from build123d import *

# Parameters (mm, degrees)
MAIN_DEPTH  = 4.7625
SKETCH2_R   = 6.35
SKETCH2_R_2 = 23.8125
HOLES_DEPTH = 67.238901193


with BuildPart() as part:
    # Sketch1 → Main (new body)
    with BuildSketch(Plane.XY):
        with BuildLine():
            Line((12.894196685, 47.360416667), (30.946072045, 22.225))
            ThreePointArc((30.946072045, 22.225), (38.1, 0), (30.946072045, -22.225))
            Line((30.946072045, -22.225), (12.894196685, -47.360416667))
            ThreePointArc((12.894196685, -47.360416667), (0, -53.975), (-12.894196685, -47.360416667))
            Line((-12.894196685, -47.360416667), (-30.946072045, -22.225))
            ThreePointArc((-30.946072045, -22.225), (-38.1, 0), (-30.946072045, 22.225))
            Line((-30.946072045, 22.225), (-12.894196685, 47.360416667))
            ThreePointArc((-12.894196685, 47.360416667), (0, 53.975), (12.894196685, 47.360416667))
        make_face()
    extrude(amount=MAIN_DEPTH)

    # Sketch2 → Holes (cut, through all)
    with BuildSketch(Plane.XY.offset(4.7625)):
        with Locations((0, 38.1)):
            Circle(SKETCH2_R)
        with Locations((0, -38.1)):
            Circle(SKETCH2_R)
        Circle(SKETCH2_R_2)
    extrude(amount=-HOLES_DEPTH, mode=Mode.SUBTRACT)


solid = part.part
The listing builds one solid part. Answer for the finished solid, in the listing's coordinates (mm). Give positions to 0.01 mm unless a question says otherwise; leave off trailing zeros. Order: outer loops, then holes, each group sorted by start corner. A loop starts at its lowest first (then second) coordinate and runs counter-clockwise, first axis right, second up. Notation, with made-up numbers: (61.25, 10.25) -> (69.25, 10.25) arc R25 ccw to (69.25, 22.25) -> close; hole circle Ø4 at (89.25, 59). An arc over 180 degrees is marked (long way). Put each result on its own line as item: value.
Item 1: A cutting plane is placed at D-D on x = 20. Give the vertices of the cut face in (y, z).
Established:
outline: (-37.47, 0) -> (-12.92, 0) -> (-12.92, 4.76) -> (-37.47, 4.76) -> close; (12.92, 0) -> (37.47, 0) -> (37.47, 4.76) -> (12.92, 4.76) -> close
Item 2: A cutting plane is placed at A-A on y = 0. Give the vertices of the cut face in (x, z).
Established:
outline: (-38.1, 0) -> (-23.81, 0) -> (-23.81, 4.76) -> (-38.1, 4.76) -> close; (23.81, 0) -> (38.1, 0) -> (38.1, 4.76) -> (23.81, 4.76) -> close
Item 3: Straight lines are drawn through the part: line 1 (X direction, y = -11, z = 2.55); line 2 (Y direction, x = -21.5, z = 2); line 3 (Y direction, x = -8, z = 1.1). For each, find the intervals that lie inside material, in ascending order.
Established:
line 1: x = -36.48 to -21.12, 21.12 to 36.48
line 2: y = -35.38 to -10.24, 10.24 to 35.38
line 3: y = -51.81 to -22.43, 22.43 to 51.81
Item 4: Given P1, Ø10, axis at x = 0, y = -38.1, coming from the +Z side; P2, Ø1.5, axis at x = -20, z = 4, coming from the +Y side, each flat-ended and moving along its own axis, determine where each tip first touches the part or whether it passes through.
Established:
P1: passes through
P2: stops at y = 38.51
Item 5: For a pull along Y with two mould halves and no side action, classify faces 1 (the face through (1, 25, 4.762)), 2 (the face through (-18.897, -14.49, 2.415)), 3 (the face through (-38.1, -0.3, 2.3)), 4 (the face through (21.794, 34.969, 2.348)) as released by +Y, released by -Y, zero draft, split by the parting line, or undercut.
Established:
face 1: zero draft
face 2: undercut
face 3: split by the parting line
face 4: released by +Y
Item 6: A cutting plane is placed at B-B on x = 0. Count the separate pieces of the cut face and the enclosed holes in it, plus the area to 3 significant figures.
Established:
separate pieces: 4
enclosed holes: 0
area: 166 mm^2
